from build123d import *

# Parameters (mm, degrees)
EXTRUDE_1_DEPTH        = 25
CUT_EXTRUDE_START      = -6
CUT_EXTRUDE_1_DEPTH    = 6
PATTERN_LINEAR_1_COUNT = 4
PATTERN_LINEAR_1_PITCH = 350
MIRROR_START           = -6
MIRROR_1_COPY_1_DEPTH  = 6
MIRROR_1_COPY_2_DEPTH  = 6
MIRROR_1_COPY_3_DEPTH  = 6
CUT_EXTRUDE_START_2    = -13
CUT_EXTRUDE_2_DEPTH    = 6


with BuildPart() as part:
    # 草图2 → 凸台-拉伸1 (new body)
    with BuildSketch(Plane.XY):
        Polygon((0, 0), (-48, -48), (1700, -48), (1748, 0), align=None)
    extrude(amount=EXTRUDE_1_DEPTH)

    # 草图3 → 切除-拉伸1 (cut)
    with BuildSketch(Plane(origin=(0, 0, 0), x_dir=(-1, 0, 0), z_dir=(0, 0, -1)).offset(CUT_EXTRUDE_START)):
        Polygon((-1402.5, 0), (-1395, -7.5), (-1355, -7.5), (-1347.5, 0), align=None)
    cut_extrude_1 = extrude(amount=-CUT_EXTRUDE_1_DEPTH, mode=Mode.SUBTRACT)

    # 阵列(线性)1: 切除-拉伸1 ×4
    with Locations(*[(-i * PATTERN_LINEAR_1_PITCH, 0, 0) for i in range(1, PATTERN_LINEAR_1_COUNT)]):
        add(cut_extrude_1, mode=Mode.SUBTRACT)

    # 镜向1: 切除-拉伸1 across plane
    add(cut_extrude_1.mirror(Plane.ZX.offset(-24)), mode=Mode.SUBTRACT)

    # 镜向1 copy 1 sketch → 镜向1 copy 1 (cut)
    with BuildSketch(Plane(origin=(-350, -48, 0), x_dir=(-1, 0, 0), z_dir=(0, 0, -1)).offset(MIRROR_START)):
        Polygon((-1402.5, 0), (-1395, 7.5), (-1355, 7.5), (-1347.5, 0), align=None)
    extrude(amount=-MIRROR_1_COPY_1_DEPTH, mode=Mode.SUBTRACT)

    # 镜向1 copy 2 sketch → 镜向1 copy 2 (cut)
    with BuildSketch(Plane(origin=(-700, -48, 0), x_dir=(-1, 0, 0), z_dir=(0, 0, -1)).offset(MIRROR_START)):
        Polygon((-1402.5, 0), (-1395, 7.5), (-1355, 7.5), (-1347.5, 0), align=None)
    extrude(amount=-MIRROR_1_COPY_2_DEPTH, mode=Mode.SUBTRACT)

    # 镜向1 copy 3 sketch → 镜向1 copy 3 (cut)
    with BuildSketch(Plane(origin=(-1050, -48, 0), x_dir=(-1, 0, 0), z_dir=(0, 0, -1)).offset(MIRROR_START)):
        Polygon((-1402.5, 0), (-1395, 7.5), (-1355, 7.5), (-1347.5, 0), align=None)
    extrude(amount=-MIRROR_1_COPY_3_DEPTH, mode=Mode.SUBTRACT)

    # 草图4 → 切除-拉伸2 (cut)
    with BuildSketch(Plane.XY.offset(25).offset(CUT_EXTRUDE_START_2)):
        Polygon((1665.5, 0), (1673, -7.5), (1740.5, -7.5), (1748, 0), align=None)
        Polygon((1665.5, -48), (1673, -40.5), (1707.5, -40.5), (1700, -48), align=None)
        Polygon((34.5, -48), (27, -40.5), (-40.5, -40.5), (-48, -48), align=None)
        Polygon((34.5, 0), (27, -7.5), (-7.5, -7.5), (0, 0), align=None)
    extrude(amount=-CUT_EXTRUDE_2_DEPTH, mode=Mode.SUBTRACT)


solid = part.part
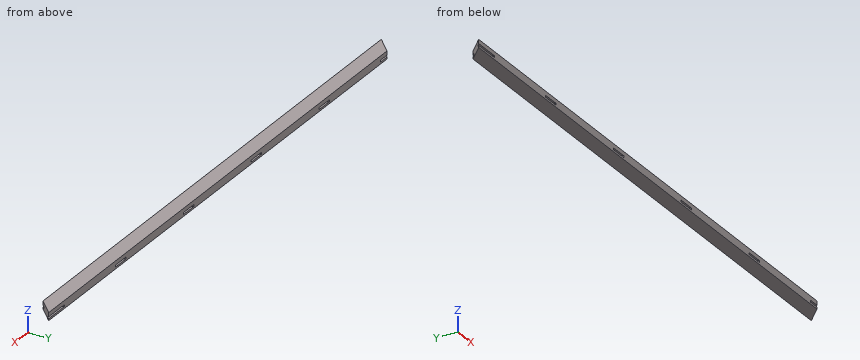
Verification items for the finished model (mm, model axes). Give positions to 0.01 mm unless a question says otherwise; leave off trailing zeros. Order: outer loops, then holes, each group sorted by start corner. A loop starts at its lowest first (then second) coordinate and runs counter-clockwise, first axis right, second up. Notation, with made-up numbers: M -8,-38.75 L 44,-38.75 A13 ccw 44,-20.75 Z; hole C 66.25,-18.75 d7. An arc over 180 degrees is marked long. Answer as a JSON object with one key per item and string values. Group by question number.
1) Cross-section at A-A (y = -29). Enter the section's corners in (x, z).
2) Scan lines: line 1 along Z through (x, y) = (1396.5, -43); line 2 along X through (y, z) = (-7.5, 5); line 3 along X through (y, z) = (-41.5, 3.25). Record each from-to range of solid material in increasing order. Write a range as [from, to].
3) Cross-section at B-B (z = 19.5). Enter the section's corners in (x, y).
4) Depth check by flat-ended pin: pin 1 Ø3 at (y, z) = (-16.5, 21) entering from -X; pin 2 Ø5 at (x, z) = (672.5, 9) entering from -Y; pin 3 Ø1.8 at (x, z) = (1694.5, 10) entering from +Y. Enter the tip coordinate at first touch or a pass-through.
Result sheet:
{
 "1": {"outline": "M -29,0 L 1719,0 L 1719,25 L -29,25 Z"},
 "2": {"line 1": "z = [0, 6], [12, 25]", "line 2": "x = [-7.5, 1740.5]", "line 3": "x = [-41.5, 1706.5]"},
 "3": {"outline": "M -48,-48 L 1700,-48 L 1748,0 L 0,0 Z"},
 "4": {"pin 1": "stops at x = -18", "pin 2": "stops at y = -40.5", "pin 3": "stops at y = -7.5"}
}
